Verification items for the finished model (mm, model axes). A direction names the side the tool comes from. Give positions to 0.01 mm unless a question says otherwise; leave off trailing zeros. Order: outer loops, then holes, each group sorted by start corner. A loop starts at its lowest first (then second) coordinate and runs counter-clockwise, first axis right, second up. Notation, with made-up numbers: (-34, 59.5) - (14, 59.5) arc R31 ccw to (14, 98.5) - close; hole circle Ø3 at (-27, -6.5). An arc over 180 degrees is marked (long way). Answer as a JSON object with one key per item and string values. Group by question number.
(1) Section check C-C (x = 5.5). Record the boundary of the cut face in (y, z).
(2) Section check A-A (z = 3.95). Record the boundary of the cut face in (x, y).
(3) Section check B-B (y = 13.7). Record the boundary of the cut face in (x, z).
(4) Access from +Z, -Z, +X, -X, +Y, -Y to the whole of each face (thin tool, end or side, straight path). Record for faces 1 (the face through (12, 7.8, 4)), 2 (the face through (12, 6, 4)), 3 (the face through (3, 7, 0)).
(5) Section check D-D (x = 15.9). Record the boundary of the cut face in (y, z).
(6) Thickness scan on line 1 (Y direction, x = 18, z = 4.75); line 2 (Z direction, x = 15.9, y = 0.8); line 3 (X direction, y = 1, z = 4.5). Record the ranges inside material, lowest first.
(7) Depth check by flat-ended pin: pin 1 Ø1 at (x, y) = (11.5, 9.5) entering from -Z; pin 2 Ø2.5 at (x, z) = (11, 3.5) entering from +Y; pin 3 Ø2.5 at (y, z) = (12, 5) entering from +X. Enter the tip coordinate at first touch or a pass-through.
(8) Mould release check, pull along Y, two halves, no side actions. Record for faces 4 (the face through (-0.336, 12.187, 3.955)), 5 (the face through (7.698, 0.887, 5.487)), 6 (the face through (8, 0, 6)), 7 (the face through (0, 17.7, 4)): +Y half, -Y half, draft (parallel to the pull), parting line (faces both ways), or undercut.
```python
from build123d import *

# Parameters (mm, degrees)
PAD_DEPTH       = 7.8
SKETCH001_R     = 1.55
POCKET_DEPTH    = 17.701
SKETCH003_R     = 1.55
POCKET001_DEPTH = 7.801


with BuildPart() as part:
    # Sketch → Pad (new body)
    with BuildSketch(Plane.XY):
        Polygon((-3.9, 17.7), (3.9, 17.7), (3.9, 7.8), (19.9, 7.8), (19.9, 6), (3.9, 6), (3.9, 1.8), (19.9, 1.8), (19.9, 0), (-3.9, 0), align=None)
    extrude(amount=PAD_DEPTH)

    # Sketch001 (on Face1 of Pad) → Pocket (cut, through all)
    with BuildSketch(Plane.XZ):
        with Locations((7.9, 3.95)):
            Circle(SKETCH001_R)
        with Locations((15.9, 3.95)):
            Circle(SKETCH001_R)
    extrude(amount=-POCKET_DEPTH, mode=Mode.SUBTRACT)

    # Sketch003 (on Face4 of Pocket) → Pocket001 (cut, through all)
    with BuildSketch(Plane.XY.offset(7.8)):
        with Locations((0, 13.7)):
            Circle(SKETCH003_R)
    extrude(amount=-POCKET001_DEPTH, mode=Mode.SUBTRACT)


solid = part.part
```
Solutions:
{
 "1": {"outline": "(0, 0) - (1.8, 0) - (1.8, 7.8) - (0, 7.8) - close; (6, 0) - (7.8, 0) - (7.8, 7.8) - (6, 7.8) - close"},
 "2": {"outline": "(-3.9, 0) - (6.35, 0) - (6.35, 1.8) - (3.9, 1.8) - (3.9, 6) - (6.35, 6) - (6.35, 7.8) - (3.9, 7.8) - (3.9, 17.7) - (-3.9, 17.7) - close; (9.45, 0) - (14.35, 0) - (14.35, 1.8) - (9.45, 1.8) - close; (9.45, 6) - (14.35, 6) - (14.35, 7.8) - (9.45, 7.8) - close; (17.45, 0) - (19.9, 0) - (19.9, 1.8) - (17.45, 1.8) - close; (17.45, 6) - (19.9, 6) - (19.9, 7.8) - (17.45, 7.8) - close; hole circle Ø3.1 at (0, 13.7)"},
 "3": {"outline": "(-3.9, 0) - (-1.55, 0) - (-1.55, 7.8) - (-3.9, 7.8) - close; (1.55, 0) - (3.9, 0) - (3.9, 7.8) - (1.55, 7.8) - close"},
 "4": {"face 1": "+Z, -Z, +X, +Y", "face 2": "+Z, -Z, +X", "face 3": "-Z, +X, -X, +Y, -Y"},
 "5": {"outline": "(0, 0) - (1.8, 0) - (1.8, 2.4) - (0, 2.4) - close; (0, 5.5) - (1.8, 5.5) - (1.8, 7.8) - (0, 7.8) - close; (6, 0) - (7.8, 0) - (7.8, 2.4) - (6, 2.4) - close; (6, 5.5) - (7.8, 5.5) - (7.8, 7.8) - (6, 7.8) - close"},
 "6": {"line 1": "y = 0 to 1.8, 6 to 7.8", "line 2": "z = 0 to 2.4, 5.5 to 7.8", "line 3": "x = -3.9 to 6.45, 9.35 to 14.45, 17.35 to 19.9"},
 "7": {"pin 1": "passes through", "pin 2": "stops at y = 7.8", "pin 3": "stops at x = 3.9"},
 "8": {"face 4": "undercut", "face 5": "draft", "face 6": "-Y half", "face 7": "+Y half"}
}
